Geometry check sheet. Reference: the model listing, model coordinates, mm. A direction names the side the tool comes from. Round coordinates to 2 decimals unless told otherwise and drop trailing zeros. Order: outer loops, then holes, each group sorted by start corner. A loop starts at its lowest first (then second) coordinate and runs counter-clockwise, first axis right, second up.
(1) Gauge pin test, flat ends, axial feed: P1, Ø1.5, axis at y = 5, z = -3, coming from the -X side; P2, Ø2, axis at y = 2.5, z = -0.5, coming from the +X side; P3, Ø4, axis at x = 30, y = 4, coming from the -Z side. Record the tip position at first contact, or that the pin passes through.
(2) Thickness scan on L1, parallel to Y at x = 31, z = 1; L2, parallel to Y at x = 16.5, z = -5; L3, parallel to X at y = 5.25, z = 1.25. Record the ranges inside material, lowest first.
(3) Draft check along Z on faces 1 (the face through (9.699, 4.056, -0.285)), 2 (the face through (5.57, 3.35, 1.01)), 3 (the face through (14.44, 5.01, -6.11)). Enter one of: pulls with the +Z half, pulls with the -Z half, needs draft (parallel to the pull), parting line crosses it, or undercut.
(4) Cross-section at C-C on y = 4. Enter the section's corners in (x, z).
(5) Cross-section at D-D on x = 16. Enter the section's corners in (y, z).
(6) Set-up check for faces 4 (the face through (4, 2, 0)), 5 (the face through (0, 4, 1)), 6 (the face through (27, 4, 0)): record each of +Z, -Z, +X, -X, +Y, -Y from which the full face is reachable in a straight line by a thin tool's end or side.
(7) Cross-section at A-A on x = 31. Enter the section's corners in (y, z).
(8) Cross-section at B-B on z = -5. Enter the section's corners in (x, y).
from build123d import *

# Parameters (mm, degrees)
BOSS_EXTRUDE1_DEPTH      = 8
M3_CLEARANCE_HOLE1_D     = 3.4
M3_CLEARANCE_HOLE1_DEPTH = 3.9
M3_CLEARANCE_HOLE1_TIP   = 1.021463052
SKETCH4_R                = 1.5
CUT_EXTRUDE1_DEPTH       = 26
FILLET1_R                = 1


with BuildPart() as part:
    # Sketch1 → Boss-Extrude1 (new body)
    with BuildSketch(Plane(origin=(0, 0, 0), x_dir=(1, 0, 0), z_dir=(0, 1, 0))):
        Polygon((0, 0), (10, 0), (10, 9), (19, 9), (19, 0), (35, 0), (35, -2), (0, -2), align=None)
    extrude(amount=BOSS_EXTRUDE1_DEPTH)

    # M3 Clearance Hole1
    with Locations(Plane(origin=(0, 0, 0), x_dir=(-1, 0, 0), z_dir=(0, 0, -1))):
        with Locations((-4, 4), (-31, 4)):
            Hole(M3_CLEARANCE_HOLE1_D / 2, depth=M3_CLEARANCE_HOLE1_DEPTH)
            with Locations((0, 0, -(M3_CLEARANCE_HOLE1_DEPTH + M3_CLEARANCE_HOLE1_TIP / 2))):  # 118° drill point
                Cone(0, M3_CLEARANCE_HOLE1_D / 2, M3_CLEARANCE_HOLE1_TIP, mode=Mode.SUBTRACT)

    # Sketch4 → Cut-Extrude1 (cut, through all)
    with BuildSketch(Plane.ZY.offset(-10)):
        with Locations((-5, 4)):
            Circle(SKETCH4_R)
    extrude(amount=-CUT_EXTRUDE1_DEPTH, mode=Mode.SUBTRACT)

    # Fillet1
    fillet1_edges = [part.edges().sort_by_distance(p)[0] for p in [
        (19, 4, 0),
        (10, 4, 0),
    ]]
    fillet(fillet1_edges, radius=FILLET1_R)


solid = part.part
Found:
1. P1: stops at x = 10
1. P2: stops at x = 35
1. P3: stops at z = 0
2. L1: y = 0 to 2.3, 5.7 to 8
2. L2: y = 0 to 2.5, 5.5 to 8
2. L3: x = 0 to 2.85, 5.15 to 29.85, 32.15 to 35
3. face 1: pulls with the -Z half
3. face 2: needs draft
3. face 3: undercut
4. outline: (0, 0) - (2.3, 0) - (2.3, 2) - (0, 2) - close; (5.7, 0) - (9, 0) arc R1 cw to (10, -1) - (10, -3.5) - (19, -3.5) - (19, -1) arc R1 cw to (20, 0) - (29.3, 0) - (29.3, 2) - (5.7, 2) - close; (10, -9) - (19, -9) - (19, -6.5) - (10, -6.5) - close; (32.7, 0) - (35, 0) - (35, 2) - (32.7, 2) - close
5. outline: (0, -9) - (8, -9) - (8, 2) - (0, 2) - close; hole circle Ø3 at (4, -5)
6. face 4: -Z, -X, +Y, -Y
6. face 5: +Z, -Z, -X, +Y, -Y
6. face 6: -Z, +X, +Y, -Y
7. outline: (0, 0) - (2.3, 0) - (2.3, 2) - (0, 2) - close; (5.7, 0) - (8, 0) - (8, 2) - (5.7, 2) - close
8. outline: (10, 0) - (19, 0) - (19, 2.5) - (10, 2.5) - close; (10, 5.5) - (19, 5.5) - (19, 8) - (10, 8) - close
